The listing builds one solid part. Answer for the finished solid, in the listing's coordinates (mm). A direction names the side the tool comes from. Give positions to 0.01 mm unless a question says otherwise; leave off trailing zeros. Order: outer loops, then holes, each group sorted by start corner. A loop starts at its lowest first (then second) coordinate and runs counter-clockwise, first axis right, second up. Notation, with made-up numbers: (46.25, 54.25) - (89.25, 54.25) arc R9 cw to (89.25, 62.25) - close; hole circle Ø9 at (-35, 84.5). An arc over 180 degrees is marked (long way). Answer as CSV lines item,"result". Start each with the question number.
1. Which of the six approach directions +Z, -Z, +X, -X, +Y, -Y give full straight-line access (tool end or side, diameter ignored) to faces 1 (the flat face through (46, 18, 11.5)), 2 (the flat face through (-47, 15, 15)), 3 (the flat face through (-6, 15, 9))?
2. Section D-D on x = 47.5 is taken. Give the vertices of the cut face in (y, z), and give its area (3 significant figures).
3. Section A-A on z = 6 is taken. Give the vertices of the cut face in (x, y), and give its area (3 significant figures).
4. Determine the mould class of faces 4 (the cylindrical face through (-34.63, 2.54, -4.26)), 5 (the cylindrical face through (22.146, 2.465, 5.324)), 6 (the flat face through (38, 12, 11)) for opening direction Z: +Z half, -Z half, draft (parallel to the pull), parting line (faces both ways), or undercut.
5. Consider line 1 along X through (y, z) = (20, 16.25); line 2 along Y through (x, z) = (47.5, 12.6); line 3 along X through (y, z) = (12, 9.25). Determine where each line is inside the solid, lowest interval first. Write a range as [from, to].
6. Section B-B on x = 20 is taken. Give the vertices of the cut face in (y, z), and give its area (4 significant figures).
7. Flat-ended cylindrical pins translate along their axes: pin 1 (6 mm diameter, centred on x = 19, y = 18.5, fed in from -Z); pin 2 (3 mm diameter, centred on x = -25, y = 9.5, fed in from -Z); pin 3 (5 mm diameter, centred on x = 47.5, y = 20, fed in from -Z); pin 4 (2 mm diameter, centred on y = 13.5, z = 3.5, fed in from +X). Find the tip coordinate at first contact, or state that the pin passes through.
8. Section C-C on x = -16 is taken. Give the vertices of the cut face in (y, z).
from build123d import *

# Parameters (mm, degrees)
SKETCH1_W            = 110
SKETCH1_H            = 30
SKETCH1_R            = 2.25
EXTRUDE_1_DEPTH      = 5
SKETCH_1_W           = 110
SKETCH_1_H           = 30
SKETCH_1_R           = 2.1
EXTRUDE_2_DEPTH      = 3
FILLET_2_R           = 10
CHAMFER1_SIZE        = 30
EXTRUDE_3_DEPTH      = 38
EXTRUDE_3_DEPTH_BACK = 38
SKETCH_3_W           = 12
SKETCH_3_H           = 15
CUT_EXTRUDE_1_DEPTH  = 26
SKETCH3_R            = 4
SKETCH3_R_2          = 2.1
BOSS_EXTRUDE1_DEPTH  = 3.5
SKETCH4_W            = 114.569016578
SKETCH4_H            = 20
CUT_EXTRUDE1_DEPTH   = 6
FILLET1_R            = 10


with BuildPart() as part:
    # Sketch1 → Бобышка-Вытянуть1 (new body)
    with BuildSketch(Plane(origin=(0, 0, 0), x_dir=(1, 0, 0), z_dir=(0, 1, 0))):
        Rectangle(SKETCH1_W, SKETCH1_H)
        with Locations((-20, -6)):
            Circle(SKETCH1_R, mode=Mode.SUBTRACT)
        with Locations((20, -6)):
            Circle(SKETCH1_R, mode=Mode.SUBTRACT)
    extrude(amount=EXTRUDE_1_DEPTH)

    # Эскиз1 → Бобышка-Вытянуть2 (add)
    with BuildSketch(Plane.XY.offset(15)):
        with Locations((0, 15)):
            Rectangle(SKETCH_1_W, SKETCH_1_H)
        with Locations((-47.5, 20)):
            Circle(SKETCH_1_R, mode=Mode.SUBTRACT)
        with Locations((47.5, 20)):
            Circle(SKETCH_1_R, mode=Mode.SUBTRACT)
    extrude(amount=EXTRUDE_2_DEPTH)

    # Скругление2
    fillet_2_edges = [part.edges().sort_by_distance(p)[0] for p in [
        (-55, 30, 16.5),
        (55, 30, 16.5),
    ]]
    fillet(fillet_2_edges, radius=FILLET_2_R)

    # Chamfer1
    chamfer1_edges = [part.edges().sort_by_distance(p)[0] for p in [
        (-55, 2.5, -15),
        (55, 2.5, -15),
    ]]
    chamfer(chamfer1_edges, length=CHAMFER1_SIZE)

    # Эскиз2 → Бобышка-Вытянуть3 (add, two sides)
    with BuildSketch(Plane(origin=(0, 0, 0), x_dir=(0, 0, -1), z_dir=(1, 0, 0))) as extrude_3_sk:
        Polygon((-15, 30), (0, 5), (-15, 5), align=None)
    extrude(amount=EXTRUDE_3_DEPTH)
    extrude(extrude_3_sk.sketch, amount=-EXTRUDE_3_DEPTH_BACK)

    # Эскиз3 → Вырез-Вытянуть1 (cut, through all)
    with BuildSketch(Plane(origin=(0, 5, 0), x_dir=(1, 0, 0), z_dir=(0, 1, 0))):
        with Locations((20, -7.5)):
            Rectangle(SKETCH_3_W, SKETCH_3_H)
        with Locations((-20, -7.5)):
            Rectangle(SKETCH_3_W, SKETCH_3_H)
        with Locations((0, -7.5)):
            Rectangle(SKETCH_3_W, SKETCH_3_H)
    extrude(amount=CUT_EXTRUDE_1_DEPTH, mode=Mode.SUBTRACT)

    # Sketch3 → Boss-Extrude1 (add)
    with BuildSketch(Plane(origin=(0, 0, 15), x_dir=(-1, 0, 0), z_dir=(0, 0, -1))):
        with Locations((-47.5, 20)):
            Circle(SKETCH3_R)
        with Locations((-47.5, 20)):
            Circle(SKETCH3_R_2, mode=Mode.SUBTRACT)
        with Locations((47.5, 20)):
            Circle(SKETCH3_R)
        with Locations((47.5, 20)):
            Circle(SKETCH3_R_2, mode=Mode.SUBTRACT)
    extrude(amount=BOSS_EXTRUDE1_DEPTH)

    # Sketch4 → Cut-Extrude1 (cut, through all)
    with BuildSketch(Plane(origin=(0, 5, 0), x_dir=(1, 0, 0), z_dir=(0, 1, 0))):
        with Locations((0, 15)):
            Rectangle(SKETCH4_W, SKETCH4_H)
    extrude(amount=-CUT_EXTRUDE1_DEPTH, mode=Mode.SUBTRACT)

    # Fillet1
    fillet1_edges = [part.edges().sort_by_distance(p)[0] for p in [
        (35, 2.5, -5),
        (-35, 2.5, -5),
    ]]
    fillet(fillet1_edges, radius=FILLET1_R)


solid = part.part
Checks:
1,face 1,"-Z, +X, +Y"
1,face 2,"-Z"
1,face 3,"-Z, +Y"
2,outline,"(0, 7.5) - (5, 7.5) - (5, 15) - (16, 15) - (16, 11.5) - (17.9, 11.5) - (17.9, 18) - (0, 18) - close; (22.1, 11.5) - (24, 11.5) - (24, 15) - (29.68, 15) - (29.68, 18) - (22.1, 18) - close"
2,area,"127 mm²"
3,outline,"(-46, 0) - (-22.25, 0) - (-22.25, 5) - (-26, 5) - (-26, 15) - (-38, 15) - (-38, 5) - (-46, 5) - close; (-17.75, 0) - (17.75, 0) - (17.75, 5) - (14, 5) - (14, 15) - (6, 15) - (6, 5) - (-6, 5) - (-6, 15) - (-14, 15) - (-14, 5) - (-17.75, 5) - close; (22.25, 0) - (46, 0) - (46, 5) - (38, 5) - (38, 15) - (26, 15) - (26, 5) - (22.25, 5) - close"
3,area,"815 mm²"
4,face 4,"-Z half"
4,face 5,"undercut"
4,face 6,"draft"
5,line 1,"x = [-55, -49.6], [-45.4, 45.4], [49.6, 55]"
5,line 2,"y = [0, 5], [16, 17.9], [22.1, 24]"
5,line 3,"x = [-38, -26], [-14, -6], [6, 14], [26, 38]"
6,outline,"(0, -5) - (5, -5) - (5, 3.75) - (0, 3.75) - close; (0, 8.25) - (5, 8.25) - (5, 15) - (30, 15) - (30, 18) - (0, 18) - close"
6,area,"167.5 mm²"
7,pin 1,"stops at z = 15"
7,pin 2,"stops at z = 2.03"
7,pin 3,"stops at z = 11.5"
7,pin 4,"passes through"
8,outline,"(0, -5) - (5, -5) - (5, 15) - (30, 15) - (30, 18) - (0, 18) - close"
